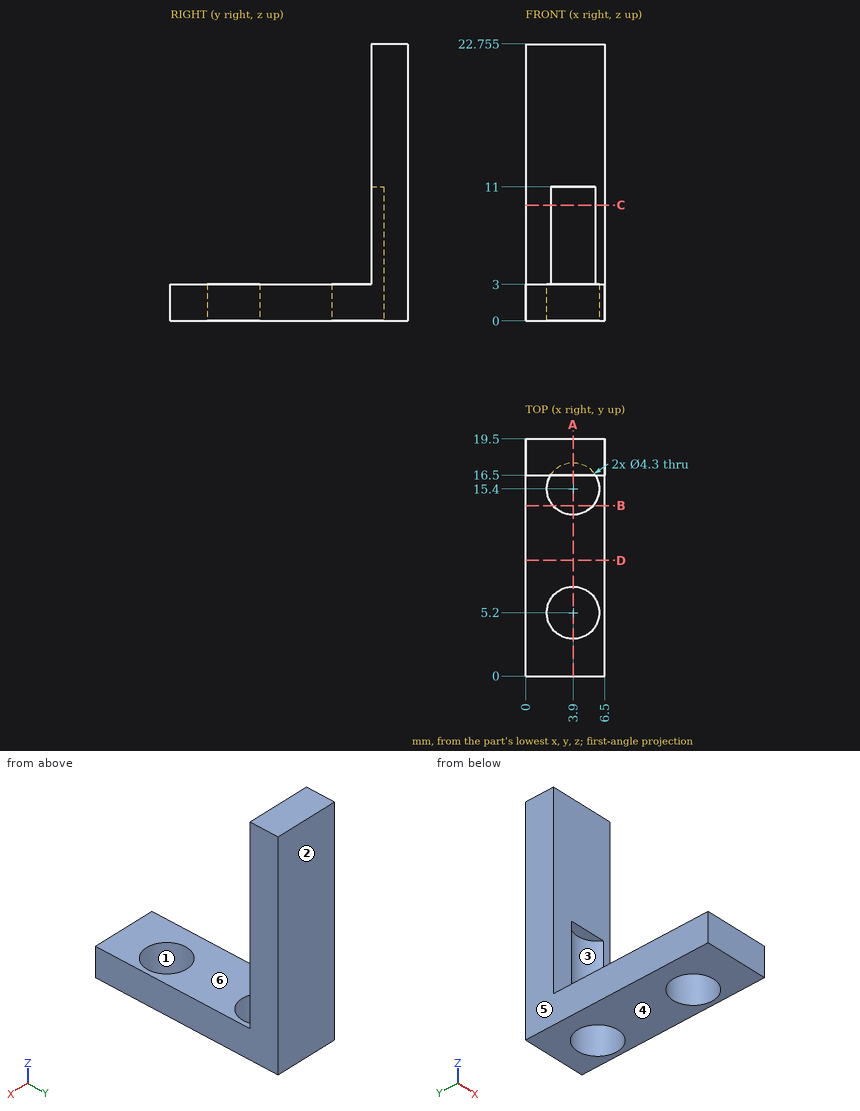
Source: three-view drawing plus pictorial views. Frame: mm from the lowest corner of the part. A direction names the side the tool comes from. Coordinates: 2 decimals unless noted, no trailing zeros. Write each loop counter-clockwise with the first axis right and the second up, starting at its lowest first coordinate (ties: lowest second). Pieces come first, ordered by that corner, then holes. Notation, with made-up numbers: (83, -7) - (104, -7) arc R20 cw to (104, 12) - close; hole circle Ø5 at (85.5, 30). An arc over 180 degrees is marked (long way). Answer as a JSON object with one key per item and string values.
Q1. Set-up query: the marked faces 5 and 6. Return all of +Z, -Z, +X, -X, +Y, -Y with unobstructed straight access to the full face (end or side cutting, diameter ignored); none if empty.
Ans:
{"face 5": "+Z, -Z, -X, +Y, -Y", "face 6": "+Z, +X, -X, -Y"}
Q2. Draft query along Y for the marked faces 1, 2, 3 and 4. Return one class per face: released by +Y, released by -Y, zero draft, split by the parting line, or undercut.
Ans:
{"face 1": "undercut", "face 2": "released by +Y", "face 3": "undercut", "face 4": "zero draft"}
Q3. Section query B-B, the plane y = 14. Output: boundary loops of the cut face in (x, z).
Ans:
{"outline": "(0, 0) - (2.27, 0) - (2.27, 3) - (0, 3) - close; (5.53, 0) - (6.5, 0) - (6.5, 3) - (5.53, 3) - close"}
Q4. Section query D-D, the plane y = 9.5. Output: boundary loops of the cut face in (x, z), plus the area to 3 significant figures.
Ans:
{"outline": "(0, 0) - (6.5, 0) - (6.5, 3) - (0, 3) - close", "area": "19.5 mm2"}
Q5. Section query C-C, the plane z = 9.5. Output: boundary loops of the cut face in (x, y).
Ans:
{"outline": "(0, 16.5) - (2.05, 16.5) arc R2.15 cw to (5.75, 16.5) - (6.5, 16.5) - (6.5, 19.5) - (0, 19.5) - close"}
Q6. Material intervals for line 1 (Y direction, x = 3.9, z = 1); line 2 (Y direction, x = 4, z = 3.5); line 3 (Z direction, x = 5.5, y = 8), sorted ascending. Write a range as [from, to].
Ans:
{"line 1": "y = [0, 3.05], [7.35, 13.25], [17.55, 19.5]", "line 2": "y = [17.55, 19.5]", "line 3": "z = [0, 3]"}
Q7. Section query A-A, the plane x = 3.9. State how many separate pieces and enclosed holes the cut face has.
Ans:
{"separate pieces": "3", "enclosed holes": "0"}
Q8. First-contact query: pin 1 Ø3 at (x, z) = (3.5, 9.5) entering from -Y; pin 2 Ø2.5 at (x, y) = (3.9, 5.2) entering from -Z; pin 3 Ø2 at (x, y) = (5, 6.5) entering from +Z. Flat tips, straight axial feed; report the tip coordinate or a pass-through.
Ans:
{"pin 1": "stops at y = 16.5", "pin 2": "passes through", "pin 3": "stops at z = 3"}
